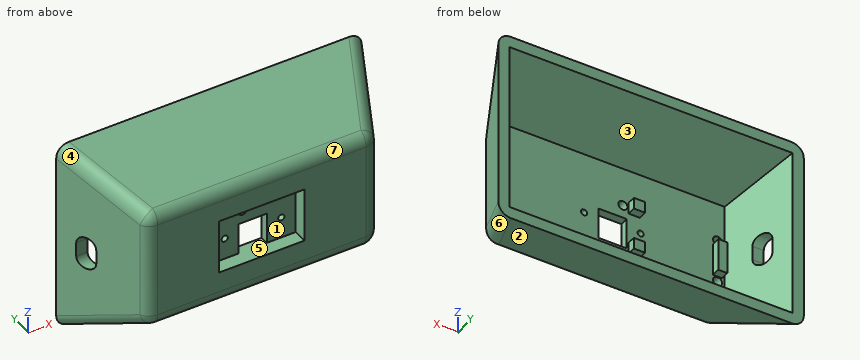
from build123d import *

# Parameters (mm, degrees)
SKETCH1_W                = 80
SKETCH1_H                = 40
BOSS_EXTRUDE1_DEPTH      = 30
BOSS_EXTRUDE1_DRAFT      = -25
SKETCH2_W                = 30.2
SKETCH2_H                = 19.2
CUT_EXTRUDE1_DEPTH       = 5
SKETCH3_W                = 99.97845949
SKETCH3_H                = 59.97845949
CUT_EXTRUDE3_DEPTH       = 22
CUT_EXTRUDE3_DRAFT       = -25
CUT_EXTRUDE4_REACH       = 70.521
SKETCH5_R                = 1.1
SKETCH5_W                = 10
SKETCH5_H                = 11
SKETCH6_R                = 1.6
PCB_HEATSETINSERTS_DEPTH = 4.75
SKETCH7_W                = 4
SKETCH7_H                = 4
SKETCH7_W_2              = 3.2
SKETCH7_H_2              = 11.55
BOSS_EXTRUDE3_DEPTH      = 3
FILLET1_R                = 5
USB_C_CUTOUT_REACH       = 102.398


with BuildPart() as part:
    # Sketch1 → Boss-Extrude1 (with draft: the straight prism first)
    with BuildSketch(Plane(origin=(0, 0, 0), x_dir=(1, 0, 0), z_dir=(0, 1, 0))):
        Rectangle(SKETCH1_W, SKETCH1_H)
    extrude(amount=BOSS_EXTRUDE1_DEPTH)
    # Boss-Extrude1: the draft: its side faces are tilted about the plane it starts from
    boss_extrude1_sides = [part.faces().sort_by_distance(p)[0] for p in [
        (-40, 15, 0),
        (0, 15, 20),
        (40, 15, 0),
        (0, 15, -20),
    ]]
    draft(boss_extrude1_sides, Plane(origin=(0, 0, 0), x_dir=(1, 0, 0), z_dir=(0, 1, 0)), BOSS_EXTRUDE1_DRAFT)

    # Sketch2 → Cut-Extrude1 (cut)
    with BuildSketch(Plane.XZ):
        Rectangle(SKETCH2_W, SKETCH2_H)
    extrude(amount=-CUT_EXTRUDE1_DEPTH, mode=Mode.SUBTRACT)


with BuildPart() as cut_extrude3_tool:
    # Sketch3 → Cut-Extrude3 (with draft: the straight prism first)
    with BuildSketch(Plane(origin=(0, 30, 0), x_dir=(1, 0, 0), z_dir=(0, 1, 0))):
        Rectangle(SKETCH3_W, SKETCH3_H)
    extrude(amount=-CUT_EXTRUDE3_DEPTH)
    # Cut-Extrude3: the draft: its side faces are tilted about the plane it starts from
    cut_extrude3_sides = [cut_extrude3_tool.faces().sort_by_distance(p)[0] for p in [
        (-49.989229745, 19, 0),
        (0, 19, 29.989229745),
        (49.989229745, 19, 0),
        (0, 19, -29.989229745),
    ]]
    draft(cut_extrude3_sides, Plane(origin=(0, 30, 0), x_dir=(1, 0, 0), z_dir=(0, 1, 0)), CUT_EXTRUDE3_DRAFT)


with BuildPart() as part_1:
    add(part.part)

    # Cut-Extrude3: cut by cut_extrude3_tool
    add(cut_extrude3_tool.part, mode=Mode.SUBTRACT)

    # Sketch5 → Cut-Extrude4 (cut, up to next)
    with BuildSketch(Plane.XZ.offset(-5), mode=Mode.PRIVATE) as cut_extrude4_sk1:
        with Locations(Location((-10, -2.1, 0), (0, 0, 270))):
            Circle(SKETCH5_R)
    cut_extrude4_tool1 = extrude(cut_extrude4_sk1.sketch, amount=-CUT_EXTRUDE4_REACH, mode=Mode.PRIVATE) & part_1.part
    # Sketch5 → Cut-Extrude4 (cut, up to next)
    with BuildSketch(Plane.XZ.offset(-5), mode=Mode.PRIVATE) as cut_extrude4_sk2:
        with Locations(Location((10, -2.1, 0), (0, 0, 270))):
            Circle(SKETCH5_R)
    cut_extrude4_tool2 = extrude(cut_extrude4_sk2.sketch, amount=-CUT_EXTRUDE4_REACH, mode=Mode.PRIVATE) & part_1.part
    # Sketch5 → Cut-Extrude4 (cut, up to next)
    with BuildSketch(Plane.XZ.offset(-5), mode=Mode.PRIVATE) as cut_extrude4_sk3:
        with Locations((-0.1, -4.1)):
            Rectangle(SKETCH5_W, SKETCH5_H)
    cut_extrude4_tool3 = extrude(cut_extrude4_sk3.sketch, amount=-CUT_EXTRUDE4_REACH, mode=Mode.PRIVATE) & part_1.part
    add(cut_extrude4_tool1.solids().sort_by_distance((-10, 5, -2.1))[0], mode=Mode.SUBTRACT)
    add(cut_extrude4_tool2.solids().sort_by_distance((10, 5, -2.1))[0], mode=Mode.SUBTRACT)
    add(cut_extrude4_tool3.solids().sort_by_distance((-0.1, 5, -4.1))[0], mode=Mode.SUBTRACT)

    # Sketch6 → PCB_HeatSetInserts (cut)
    with BuildSketch(Plane(origin=(0, 8, 0), x_dir=(1, 0, 0), z_dir=(0, 1, 0))):
        with Locations(Location((-37.190461265, -5.98, 0), (0, 0, 270))):
            Circle(SKETCH6_R)
        with Locations(Location((-37.190461265, 9.27, 0), (0, 0, 270))):
            Circle(SKETCH6_R)
        with Locations(Location((-3.730461265, -5.98, 0), (0, 0, 270))):
            Circle(SKETCH6_R)
    extrude(amount=-PCB_HEATSETINSERTS_DEPTH, mode=Mode.SUBTRACT)

    # Sketch7 → Boss-Extrude3 (add)
    with BuildSketch(Plane(origin=(0, 8, 0), x_dir=(1, 0, 0), z_dir=(0, 1, 0))):
        with Locations((-7.730461265, -5.7)):
            Rectangle(SKETCH7_W, SKETCH7_H)
        with Locations((-37.190461265, 1.645)):
            Rectangle(SKETCH7_W_2, SKETCH7_H_2)
        with Locations((-7.730461265, 9.3)):
            Rectangle(SKETCH7_W, SKETCH7_H)
    extrude(amount=BOSS_EXTRUDE3_DEPTH)

    # Fillet1
    fillet1_edges = [part_1.edges().sort_by_distance(p)[0] for p in [
        (0, 0, 20),
        (-40, 0, 0),
        (0, 0, -20),
        (40, 0, 0),
        (46.994614872, 15, 26.994614872),
        (-46.994614872, 15, 26.994614872),
        (-46.994614872, 15, -26.994614872),
        (46.994614872, 15, -26.994614872),
    ]]
    fillet(fillet1_edges, radius=FILLET1_R)

    # USB-C Cutout: up to this plane
    usb_c_cutout_end = Plane(origin=(-40, 0, -20), z_dir=(-0.9063077870366496, -0.4226182617407003, 0))
    # Sketch10 → USB-C Cutout (cut, up to the surface)
    with BuildSketch(Plane(origin=(-35.590461265, 0, 0), x_dir=(0, 0, -1), z_dir=(1, 0, 0)), mode=Mode.PRIVATE) as usb_c_cutout_sk1:
        with BuildLine():
            Line((-0.855, 23.5), (4.145, 23.5))
            ThreePointArc((4.145, 23.5), (7.395, 20.25), (4.145, 17))
            Line((4.145, 17), (-0.855, 17))
            ThreePointArc((-0.855, 17), (-4.105, 20.25), (-0.855, 23.5))
        make_face()
    usb_c_cutout_tool1 = split(extrude(usb_c_cutout_sk1.sketch, amount=-USB_C_CUTOUT_REACH, mode=Mode.PRIVATE), bisect_by=usb_c_cutout_end, keep=Keep.BOTH, mode=Mode.PRIVATE)
    add(usb_c_cutout_tool1.solids().sort_by_distance((-35.590461, 20.25, -1.645))[0], mode=Mode.SUBTRACT)


solid = part_1.part
CAD build for the part. Positions are in the model's coordinates, mm. Face numbers are marked on the shaded views. A direction names the side the tool comes from. Give positions to 0.01 mm unless a question says otherwise; leave off trailing zeros. Write each loop counter-clockwise with the first axis right and the second up, starting at its lowest first coordinate (ties: lowest second). Pieces come first, ordered by that corner, then holes. Notation, with made-up numbers: (-22, 72) -> (25, 72) arc R26 cw to (25, 104) -> close; hole circle Ø5 at (-39.5, 3.25). An arc over 180 degrees is marked (long way). Return JSON: item names as keys, results as strings.
Item 1: Drill centre lines: probe 1 along X at (y, z) = (6.75, 5.98); probe 2 along X at (y, z) = (9, -3); probe 3 along Y at (x, z) = (-6.5, 7). Where is each one in solid material? Low to high.
Answer below:
{"probe 1": "x = -43.15 to -38.79, -35.59 to -5.33, -2.13 to 43.15", "probe 2": "x = -44.2 to -40.2, -38.79 to -35.59, 40.2 to 44.2", "probe 3": "y = 5 to 11"}
Item 2: Band-saw the part on B-B (z = 5.98). List the corners of the cut face in (x, y), then the cut area to 3 significant figures.
Answer below:
{"outline": "(-53.99, 30) -> (-41.35, 2.89) arc R5 ccw to (-36.81, 0) -> (-15.1, 0) -> (-15.1, 5) -> (-5.33, 5) -> (-5.33, 8) -> (-5.73, 8) -> (-5.73, 11) -> (-9.73, 11) -> (-9.73, 8) -> (-35.59, 8) -> (-35.59, 3.25) -> (-38.79, 3.25) -> (-38.79, 8) -> (-39.73, 8) -> (-49.99, 30) -> close; (-2.13, 5) -> (15.1, 5) -> (15.1, 0) -> (36.81, 0) arc R5 ccw to (41.35, 2.89) -> (53.99, 30) -> (49.99, 30) -> (39.73, 8) -> (-2.13, 8) -> close", "area": "679 mm2"}
Item 3: Two-plate mould, pull along X, no slides. Class the marked faces 4, 5, 6 and 7: +X half, -X half, draft (parallel to the pull), parting line (faces both ways), or undercut.
Answer below:
{"face 4": "-X half", "face 5": "undercut", "face 6": "+X half", "face 7": "draft"}
Item 4: Band-saw the part on C-C (x = -13.5). List the corners of the cut face in (y, z), then the cut area to 3 significant figures.
Answer below:
{"outline": "(0, -16.81) arc R5 ccw to (2.89, -21.35) -> (30, -33.99) -> (30, -29.99) -> (8, -19.73) -> (8, 19.73) -> (30, 29.99) -> (30, 33.99) -> (2.89, 21.35) arc R5 ccw to (0, 16.81) -> (0, 9.6) -> (5, 9.6) -> (5, -9.6) -> (0, -9.6) -> close", "area": "426 mm2"}
Item 5: Drop flat-ended pins along their axis: pin 1 (1.5 mm diameter, centred on y = 7, z = -4, fed in from -X); pin 2 (2 mm diameter, centred on y = 23, z = -9.5, fed in from +X); pin 3 (12 mm diameter, centred on x = -9, y = 21.5, fed in from -Z); pin 4 (4 mm diameter, centred on x = -37.19, z = 5.98, fed in from -Y). Give the stop position or say it passes through.
Answer below:
{"pin 1": "stops at x = -43.61", "pin 2": "stops at x = 51.19", "pin 3": "stops at z = -32.82", "pin 4": "stops at y = 0"}
Item 6: Tool access for the marked faces 1, 2 and 3: list every direction of +Z, -Z, +X, -X, +Y, -Y with a clear straight run to the whole face (end or side of a thin tool).
Answer below:
{"face 1": "-Y", "face 2": "-Z, +X, -X, -Y", "face 3": "+Y"}
Item 7: Band-saw the part on A-A (x = 10). List the corners of the cut face in (y, z), then the cut area to 3 significant figures.
Answer below:
{"outline": "(0, -16.81) arc R5 ccw to (2.89, -21.35) -> (30, -33.99) -> (30, -29.99) -> (8, -19.73) -> (8, -3.2) -> (5, -3.2) -> (5, -9.6) -> (0, -9.6) -> close; (0, 9.6) -> (5, 9.6) -> (5, -1) -> (8, -1) -> (8, 19.73) -> (30, 29.99) -> (30, 33.99) -> (2.89, 21.35) arc R5 ccw to (0, 16.81) -> close", "area": "420 mm2"}
